Can you work these out from the drawing? Everything is in mm from the part's minimum corner. A direction names the side the tool comes from. Round coordinates to 2 decimals unless told otherwise and drop trailing zeros. Loops run counter-clockwise (first coordinate to the right, second up) from the corner with the lowest first, then second, coordinate; pieces in that order, holes last. Notation, with made-up numbers: M -25.5,5.25 L 23.5,5.25 A18 cw 23.5,27.25 Z; hole C -5,72 d11. An arc over 180 degrees is marked long. Use a Markdown table: item, result.
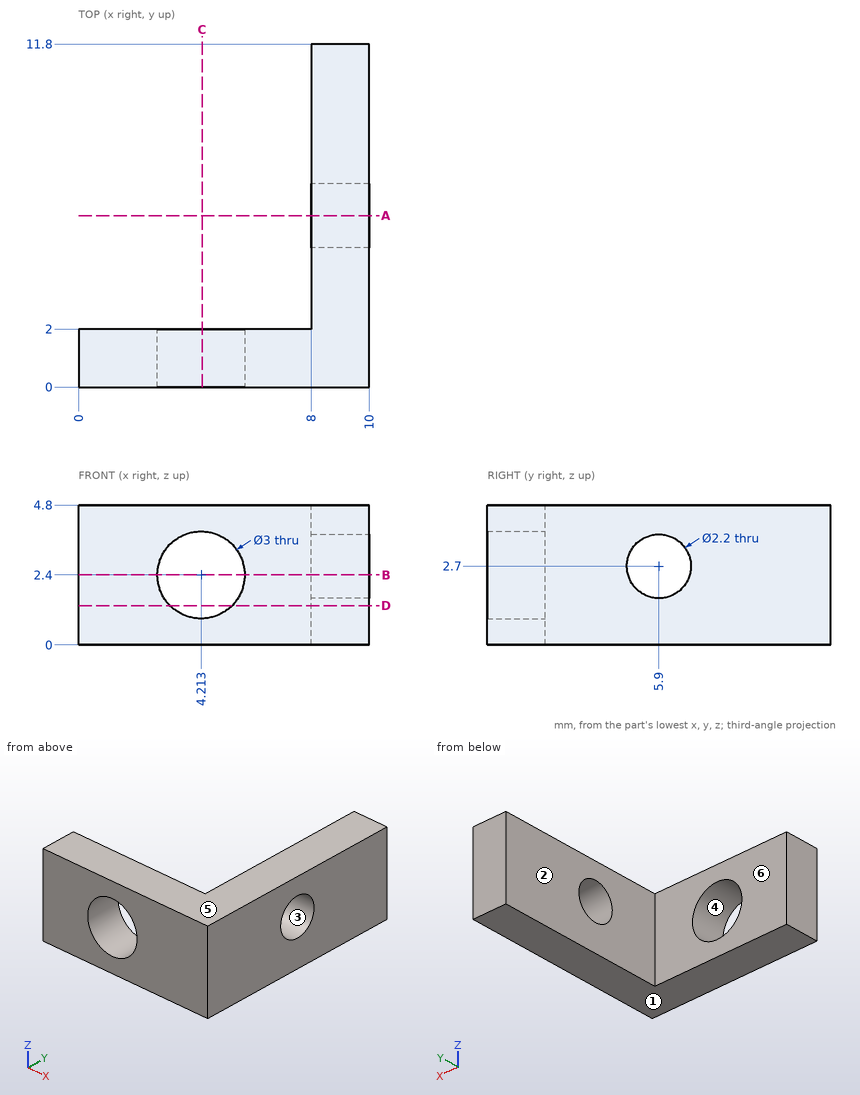
1. Imagine slicing it at B-B, the plane z = 2.4. Write out the boundary of the cut face in (x, y).
Answer sheet:
| item | result |
|---|---|
| outline | M 0,0 L 2.71,0 L 2.71,2 L 0,2 Z; M 5.71,0 L 10,0 L 10,4.84 L 8,4.84 L 8,2 L 5.71,2 Z; M 8,6.96 L 10,6.96 L 10,11.8 L 8,11.8 Z |
2. Imagine slicing it at A-A, the plane y = 5.9. Write out the boundary of the cut face in (x, z).
Answer sheet:
| item | result |
|---|---|
| outline | M 8,0 L 10,0 L 10,1.6 L 8,1.6 Z; M 8,3.8 L 10,3.8 L 10,4.8 L 8,4.8 Z |
3. Which directions (+Z, -Z, +X, -X, +Y, -Y) give clear straight access to the entire face, cutting with the end or side of a thin tool? Please do the marked faces 5 and 6.
Answer sheet:
| item | result |
|---|---|
| face 5 | +Z, +X, -X, +Y, -Y |
| face 6 | +Z, -Z, -X, +Y |
4. Imagine slicing it at C-C, the plane x = 4.25. Write out the boundary of the cut face in (y, z).
Answer sheet:
| item | result |
|---|---|
| outline | M 0,0 L 2,0 L 2,0.9 L 0,0.9 Z; M 0,3.9 L 2,3.9 L 2,4.8 L 0,4.8 Z |
5. I need wall thicknesses on probe 1 along Y at (x, z) = (9.2, 2.7); probe 2 along X at (y, z) = (0.5, 2.4); probe 3 along Y at (x, z) = (5.75, 4.3). Which ranges of each line are inside material? Lowest first, please. Write a range as from..to.
Answer sheet:
| item | result |
|---|---|
| probe 1 | 0..4.8, 7..11.8 |
| probe 2 | 0..2.71, 5.71..10 |
| probe 3 | 0..2 |
6. Imagine slicing it at D-D, the plane z = 1.35. Write out the boundary of the cut face in (x, y) (1 decimal).
Answer sheet:
| item | result |
|---|---|
| outline | M 0,0 L 3.1,0 L 3.1,2 L 0,2 Z; M 5.3,0 L 10,0 L 10,11.8 L 8,11.8 L 8,2 L 5.3,2 Z |
7. We'd pull the mould along Z, two halves only. Please class the marked faces 1, 2, 3 and 4: +Z half, -Z half, draft (parallel to the pull), parting line (faces both ways), or undercut.
Answer sheet:
| item | result |
|---|---|
| face 1 | -Z half |
| face 2 | draft |
| face 3 | undercut |
| face 4 | undercut |
8. For pin 1 Ø1.5 at (x, z) = (7.5, 0.5) entering from -Y, with a flat end and sliding along its axis, tell me the tip position at first contact or that it passes through.
Answer sheet:
| item | result |
|---|---|
| pin 1 | y = 0 |
